Here's how the part is built. I have some questions about the finished solid (model axes, mm). A direction names the side the tool comes from. Coordinates: 2 decimals unless noted, no trailing zeros. Order: outer loops, then holes, each group sorted by start corner. A loop starts at its lowest first (then second) coordinate and runs counter-clockwise, first axis right, second up. Notation, with made-up numbers: (7, -2.75) - (43, -2.75) arc R20 ccw to (43, 4.25) - close; hole circle Ø9 at (35.25, -9). An arc over 180 degrees is marked (long way). Answer as CSV lines item,"result". Start each with the question number.
Item 1: I need wall thicknesses on line 1 (X direction, y = 14.5, z = 0); line 2 (Z direction, x = 0, y = 20.5); line 3 (Z direction, x = -28, y = 31.5). Which ranges of each line are inside material? Lowest first, please.
Item 2: I'm going to push flat-ended pins straight in: pin 1 (12 mm diameter, centred on x = -14.5, y = 22, fed in from -Z); pin 2 (2 mm diameter, centred on y = 17, z = -16.5, fed in from +X); pin 3 (4 mm diameter, centred on x = 0, z = 0, fed in from +Y); pin 4 (5 mm diameter, centred on x = -18.5, y = 32, fed in from +Z). Where does each tip first touch, or does it pass through?
Item 3: Imagine slicing it at A-A on z = 0. List the corners of the cut face in (x, y) for me.
Item 4: We'd pull the mould along Z, two halves only. Please class faces 3 (the face through (19.873, 25.35, 10.846)), 4 (the face through (-8.71, 25.35, 20.9)), 5 (the face through (-10.076, 24.65, 30.899)), 6 (the face through (21.77, 24.65, -24.13)): pulls with the +Z half, pulls with the -Z half, needs draft (parallel to the pull), parting line crosses it, or undercut.
Item 5: Imagine slicing it at B-B on z = 14. Count the separate pieces of the cut face and the enclosed holes in it, and give its area (3 significant figures).
Item 6: On a 3-axis mill with a long thin cutter (end or side, diameter ignored), from which of +Z, -Z, +X, -X, +Y, -Y can I reach the whole of each face in a straight line? I mean faces 1 (the face through (-16.28, 24.65, 28.13)), 2 (the face through (8.605, 25.35, 20.638)). Say none if no direction works.
from build123d import *

# Parameters (mm, degrees)
SKETCH1_R               = 32.5
BOSS_EXTRUDE1_DEPTH     = 50
CUT_EXTRUDE1_DEPTH      = 68.915388536
CIRPATTERN1_COUNT       = 30
CUT_EXTRUDE2_DEPTH      = 68.909114756
CUT_EXTRUDE2_DEPTH_BACK = 68.909114756
SKETCH3_R               = 2.5


with BuildPart() as part:
    # Sketch1 → Boss-Extrude1 (new body)
    with BuildSketch(Plane(origin=(0, 0, 0), x_dir=(1, 0, 0), z_dir=(0, 1, 0))):
        with Locations(Location((0, 0, 0), (0, 0, 270))):
            Circle(SKETCH1_R)
    extrude(amount=BOSS_EXTRUDE1_DEPTH)

    # Sketch2 → Cut-Extrude1 (cut, symmetric)
    with BuildSketch(Plane(origin=(0, 50, 0), x_dir=(1, 0, 0), z_dir=(0, 1, 0))):
        Polygon((-6.928301674, 188.527455376), (-0.923110544, 32.486887615), (-0.153919032, 12.5), (0.153919032, 12.5), (0.923110544, 32.486887615), (6.928301674, 188.527455376), (6.928301674, 500.839614011), (-6.928301674, 500.839614011), align=None)
    cut_extrude1 = extrude(amount=CUT_EXTRUDE1_DEPTH, both=True, mode=Mode.SUBTRACT)

    # CirPattern1: Cut-Extrude1 ×30 about axis
    cirpattern1_axis = Axis((0, 50, 0), (0, 1, 0))
    for i in range(1, CIRPATTERN1_COUNT):
        add(cut_extrude1.rotate(cirpattern1_axis, i * 360 / CIRPATTERN1_COUNT), mode=Mode.SUBTRACT)

    # Sketch3 → Cut-Extrude2 (cut, two sides: drawn at the far end of the back side and taken through both)
    with BuildSketch(Plane(origin=(0, 50, 0), x_dir=(1, 0, 0), z_dir=(0, 1, 0)).offset(-CUT_EXTRUDE2_DEPTH_BACK)):
        with Locations(Location((0, 0, 0), (0, 0, 270))):
            Circle(SKETCH3_R)
    extrude(amount=CUT_EXTRUDE2_DEPTH + CUT_EXTRUDE2_DEPTH_BACK, mode=Mode.SUBTRACT)


solid = part.part
Responses:
1,line 1,"x = -32.5 to -2.5, 2.5 to 32.5"
1,line 2,"z = -12.5 to -2.5, 2.5 to 12.5"
1,line 3,"z = -15.13 to -9.96, -8.26 to -3.71, -2.19 to 2.19, 3.71 to 8.26, 9.96 to 15.13"
2,pin 1,"stops at z = -31.37"
2,pin 2,"stops at x = 27.67"
2,pin 3,"passes through"
2,pin 4,"stops at z = 28.29"
3,outline,"(-32.5, 0) - (-2.5, 0) - (-2.5, 50) - (-32.5, 50) - close; (2.5, 0) - (32.5, 0) - (32.5, 50) - (2.5, 50) - close"
4,face 3,"undercut"
4,face 4,"undercut"
4,face 5,"pulls with the +Z half"
4,face 6,"pulls with the -Z half"
5,separate pieces,"12"
5,enclosed holes,"0"
5,area,"2,280 mm^2"
6,face 1,"+Z, -X, +Y, -Y"
6,face 2,"+Y, -Y"
